```python
from build123d import *

# Parameters (mm, degrees)
SKETCH_1_W      = 15
SKETCH_1_H      = 1
EXTRUDE_1_DEPTH = 0.5
SKETCH_2_W      = 1
SKETCH_2_H      = 1
EXTRUDE_2_DEPTH = 8
FILLET_1_R      = 2


with BuildPart() as part:
    # Эскиз1 → Бобышка-Вытянуть1 (new, symmetric)
    with BuildSketch(Plane(origin=(0, 0, 0), x_dir=(1, 0, 0), z_dir=(0, 1, 0))):
        Rectangle(SKETCH_1_W, SKETCH_1_H)
    extrude(amount=EXTRUDE_1_DEPTH, both=True)

    # Эскиз2 → Бобышка-Вытянуть2 (add)
    with BuildSketch(Plane.XZ.offset(0.5)):
        with Locations((-7, 0)):
            Rectangle(SKETCH_2_W, SKETCH_2_H)
        with Locations((7, 0)):
            Rectangle(SKETCH_2_W, SKETCH_2_H)
    extrude(amount=EXTRUDE_2_DEPTH)

    # Скругление1
    fillet_1_edges = [part.edges().sort_by_distance(p)[0] for p in [
        (-7.5, 0.5, 0),
        (-6.5, -0.5, 0),
        (6.5, -0.5, 0),
        (7.5, 0.5, 0),
    ]]
    fillet(fillet_1_edges, radius=FILLET_1_R)


solid = part.part
```
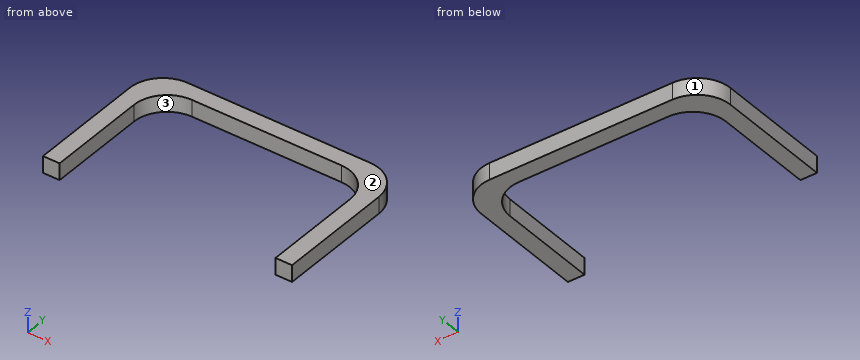
Design review of the part built by this model. Coordinates are the model's own, in mm. Face numbers are marked on the shaded views. Coordinates: 2 decimals unless noted, no trailing zeros. Loops run counter-clockwise (first coordinate to the right, second up) from the corner with the lowest first, then second, coordinate; pieces in that order, holes last.
Q1. The part is to be moulded in two halves that separate along X. For the marked faces 1, 2 and 3, say which applies: +X half, -X half, draft (parallel to the pull), parting line (faces both ways), or undercut.
Reported:
face 1: -X half
face 2: draft
face 3: undercut
Q2. We need section A-A on y = -7. State the section outline as (x, z) points.
Reported:
outline: (-7.5, -0.5) - (-6.5, -0.5) - (-6.5, 0.5) - (-7.5, 0.5) - close; (6.5, -0.5) - (7.5, -0.5) - (7.5, 0.5) - (6.5, 0.5) - close
Q3. To check wall thickness, follow line 1 (X direction, y = -4, z = 0.15); line 2 (Y direction, x = -0.75, z = 0.1); line 3 (X direction, y = -0.75, z = -0.2). State the ranges of each line that lie inside material, in increasing order.
Reported:
line 1: x = -7.5 to -6.5, 6.5 to 7.5
line 2: y = -0.5 to 0.5
line 3: x = -7.35 to -5.47, 5.47 to 7.35
Q4. We need section C-C on x = 3. State the section outline as (y, z) points, and give its area (3 significant figures).
Reported:
outline: (-0.5, -0.5) - (0.5, -0.5) - (0.5, 0.5) - (-0.5, 0.5) - close
area: 1.00 mm2
Q5. For pin 1 (0.5 mm diameter, centred on x = 1, z = 0, fed in from -Y), flat-tipped, find the tip position at first contact; note if it passes through.
Reported:
pin 1: stops at y = -0.5
Q6. We need section B-B on z = -0.05. State the section outline as (x, y) points.
Reported:
outline: (-7.5, -8.5) - (-6.5, -8.5) - (-6.5, -2.5) arc R2 cw to (-4.5, -0.5) - (4.5, -0.5) arc R2 cw to (6.5, -2.5) - (6.5, -8.5) - (7.5, -8.5) - (7.5, -1.5) arc R2 ccw to (5.5, 0.5) - (-5.5, 0.5) arc R2 ccw to (-7.5, -1.5) - close
Q7. We need section D-D on y = -2.25. State the section outline as (x, z) points.
Reported:
outline: (-7.5, -0.5) - (-6.48, -0.5) - (-6.48, 0.5) - (-7.5, 0.5) - close; (6.48, -0.5) - (7.5, -0.5) - (7.5, 0.5) - (6.48, 0.5) - close
